from build123d import *

# Parameters (mm, degrees)
PAD_DEPTH    = 32
POCKET_DEPTH = 30


with BuildPart() as part:
    # Sketch → Pad (new body)
    with BuildSketch(Plane.XY):
        with BuildLine():
            Line((68, 11.919847), (68, 52.484752))
            ThreePointArc((68, 52.484752), (65.982797, 59.902078), (60.486868, 65.276144))
            ThreePointArc((60.486868, 65.276144), (31.248603, 77.004779), (0, 81))
            Line((0, 81), (0, 7.903371))
            ThreePointArc((51.786627, 0), (26.193119, 5.916155), (0, 7.903371))
            ThreePointArc((51.786627, 0), (62.908928, 1.858085), (68, 11.919847))
        make_face()
        with BuildLine():
            Line((56.278101, 57.375088), (51.762611, 47.798227))
            ThreePointArc((51.762611, 47.798227), (54.509093, 42.183801), (59.387684, 46.090756))
            Line((59.387684, 56.678764), (59.387684, 46.090756))
            ThreePointArc((59.387684, 56.678764), (58.111713, 58.27206), (56.278101, 57.375088))
        make_face(mode=Mode.SUBTRACT)
    pad = extrude(amount=PAD_DEPTH)

    # Sketch001 → Pocket (cut)
    with BuildSketch(Plane.XY.offset(32)):
        with BuildLine():
            ThreePointArc((43.162552, 57.77313), (21.99443, 64.319264), (0, 67))
            Line((0, 67), (0, 40))
            ThreePointArc((0, 40), (5.362658, 40.184337), (10.7, 40.736478))
            ThreePointArc((12.666923, 37.969749), (12.125079, 39.667069), (10.7, 40.736478))
            Line((12.666923, 31.822003), (12.666923, 37.969749))
            ThreePointArc((12.666923, 31.822003), (13.078436, 30.695708), (14.119116, 30.1))
            ThreePointArc((14.119116, 30.1), (23.572379, 29.366387), (33, 30.377498))
            ThreePointArc((36.047549, 27.450542), (35.147342, 29.563278), (33, 30.377498))
            Line((36.047549, 19.83336), (36.047549, 27.450542))
            ThreePointArc((36.047549, 19.83336), (36.499771, 18.620595), (37.635625, 18))
            ThreePointArc((37.635625, 18), (45.958329, 17.472818), (54.258916, 18.276295))
            ThreePointArc((54.258916, 18.276295), (54.788961, 18.583293), (54.998194, 19.158982))
            Line((54.998194, 28.871338), (54.998194, 19.158982))
            ThreePointArc((54.998194, 28.871338), (52.927452, 32.928287), (48.905587, 35.066376))
            ThreePointArc((44.75866, 49.161724), (42.505536, 40.841145), (48.905587, 35.066376))
            ThreePointArc((44.75866, 49.161724), (46.308059, 53.902523), (43.162552, 57.77313))
        make_face()
    pocket = extrude(amount=-POCKET_DEPTH, mode=Mode.SUBTRACT)

    # Mirrored: Pad, Pocket across Sketch001 V_Axis
    add(pad.mirror(Plane(origin=(0, 0, 32), x_dir=(0, 0, 1), z_dir=(1, 0, 0))))
    add(pocket.mirror(Plane(origin=(0, 0, 32), x_dir=(0, 0, 1), z_dir=(1, 0, 0))), mode=Mode.SUBTRACT)


solid = part.part
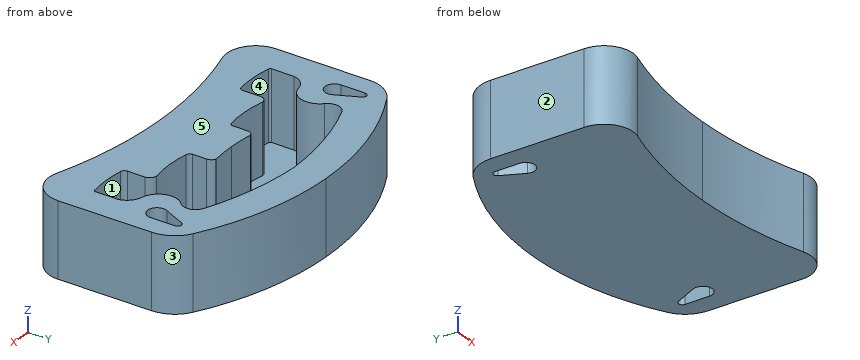
Design review of the part built by this model. Coordinates are the model's own, in mm. Face numbers are marked on the shaded views. A direction names the side the tool comes from. Coordinates: 2 decimals unless noted, no trailing zeros. Order: outer loops, then holes, each group sorted by start corner. A loop starts at its lowest first (then second) coordinate and runs counter-clockwise, first axis right, second up.
Item 1: Take a section at A-A, the plane y = 51. Write out the cut boundary in (x, z).
Item 2: Take a section at B-B, the plane x = 4. Write out the cut boundary in (y, z).
Item 3: Take a section at C-C, the plane x = -18. Write out the cut boundary in (y, z), then the cut area to 3 significant figures.
Item 4: For pin 1 Ø12 at (x, y) = (-17, 40.5) entering from -Z; pin 2 Ø1 at (x, z) = (51.5, 6.5) entering from +Y; pin 3 Ø8 at (y, z) = (58.5, 4.5) entering from -X; pin 4 Ø4 at (x, z) = (-41, 24.5) entering from +Y, all flat-tipped, find the tip position at first contact; note any pin that passes through.
Item 5: For line 1 (X direction, y = 24, z = 8); line 2 (X direction, y = 52, z = 27); line 3 (X direction, y = 54.5, z = 29), list the stretches that pass through material, from the lowest coordinate up.
Item 6: Take a section at D-D, the plane z = 13. Count the separate pieces of the cut face and the enclosed holes in it, then the cut area to 3 significant figures.
Item 7: For the marked faces 1 and 2, list the 3-axis set-ups (+Z, -Z, +X, -X, +Y, -Y) from which the entire face can be reached by the end or side of a thin tool; tool diameter is ignored.
Item 8: The part is to be moulded in two halves that separate along X. For the marked faces 3, 4 and 5, say which applies: pulls with the +X half, pulls with the -X half, needs draft (parallel to the pull), parting line crosses it, or undercut.
The answers:
1. outline: (-68, 0) - (-59.39, 0) - (-59.39, 32) - (-68, 32) - close; (-53.27, 0) - (53.27, 0) - (53.27, 32) - (46.02, 32) - (46.02, 2) - (-46.02, 2) - (-46.02, 32) - (-53.27, 32) - close; (59.39, 0) - (68, 0) - (68, 32) - (59.39, 32) - close
2. outline: (7.86, 0) - (80.94, 0) - (80.94, 32) - (66.81, 32) - (66.81, 2) - (40.1, 2) - (40.1, 32) - (7.86, 32) - close
3. outline: (6.97, 0) - (79.69, 0) - (79.69, 32) - (65.1, 32) - (65.1, 2) - (29.59, 2) - (29.59, 32) - (6.97, 32) - close
3. area: 1,260 mm2
4. pin 1: stops at z = 0
4. pin 2: stops at y = 70.05
4. pin 3: stops at x = -67.86
4. pin 4: stops at y = 74.72
5. line 1: x = -68 to -55, -36.05 to 36.05, 55 to 68
5. line 2: x = -68 to -59.39, -53.74 to -46.31, 46.31 to 53.74, 59.39 to 68
5. line 3: x = -67.86 to -59.39, -54.92 to -46.16, 46.16 to 54.92, 59.39 to 67.86
6. separate pieces: 1
6. enclosed holes: 3
6. area: 6,050 mm2
7. face 1: +Z
7. face 2: +Z, -Z, -X, +Y, -Y
8. face 3: pulls with the +X half
8. face 4: undercut
8. face 5: needs draft
